Geometry check sheet. Reference: the model listing, model coordinates, mm. Give positions to 0.01 mm unless a question says otherwise; leave off trailing zeros. Write each loop counter-clockwise with the first axis right and the second up, starting at its lowest first coordinate (ties: lowest second). Pieces come first, ordered by that corner, then holes.
(1) Cross-section at B-B (z = -70). Record the boundary of the cut face in (x, y).
(2) Depth check by flat-ended pin: P1, Ø4, axis at y = 188, z = -296, coming from the -X side. Enter the tip coordinate at first touch or a pass-through.
(3) Cross-section at A-A (y = 65). Record the boundary of the cut face in (x, z).
(4) Thickness scan on line 1 along Z through (x, y) = (0.6, 265.06); line 2 along Z through (x, y) = (0.55, 188); line 3 along Y through (x, z) = (0.5, -314). Record the ranges inside material, lowest first.
(5) Cross-section at C-C (x = 0.8). Count the separate pieces of the cut face and the enclosed holes in it, and give its area (3 significant figures).
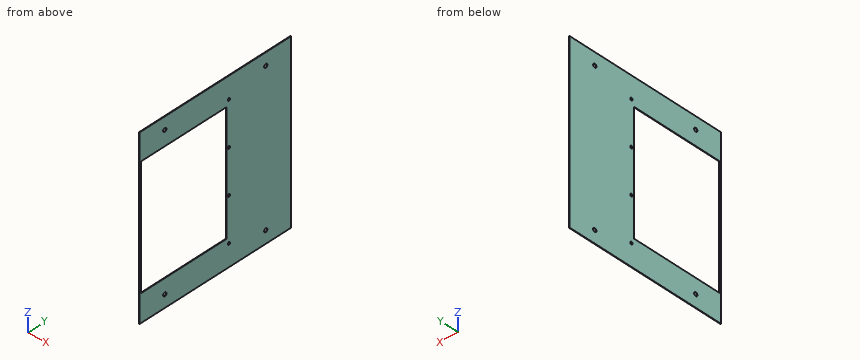
```python
from build123d import *

# Parameters (mm, degrees)
SKETCH1_W           = 338
SKETCH1_H           = 318
SKETCH1_R           = 3.5
BOSS_EXTRUDE1_DEPTH = 1
SKETCH2_R           = 2.5
SKETCH2_W           = 232.5
SKETCH2_H           = 180
CUT_EXTRUDE1_DEPTH  = 2


with BuildPart() as part:
    # Sketch1 → Boss-Extrude1 (new body)
    with BuildSketch(Plane(origin=(0, 0, 0), x_dir=(0, 0, -1), z_dir=(1, 0, 0))):
        with Locations((169, 159)):
            Rectangle(SKETCH1_W, SKETCH1_H)
        with Locations((24, 265.06)):
            Circle(SKETCH1_R, mode=Mode.SUBTRACT)
        with Locations((314, 265.06)):
            Circle(SKETCH1_R, mode=Mode.SUBTRACT)
        with Locations((314, 52.94)):
            Circle(SKETCH1_R, mode=Mode.SUBTRACT)
        with Locations((24, 52.94)):
            Circle(SKETCH1_R, mode=Mode.SUBTRACT)
    extrude(amount=BOSS_EXTRUDE1_DEPTH)

    # Sketch2 → Cut-Extrude1 (cut, through all)
    with BuildSketch(Plane.ZY):
        with Locations((-296, 188)):
            Circle(SKETCH2_R)
        with Locations((-211.333333333, 188)):
            Circle(SKETCH2_R)
        with Locations((-126.666666667, 188)):
            Circle(SKETCH2_R)
        with Locations((-42, 188)):
            Circle(SKETCH2_R)
        with Locations((-169, 93)):
            Rectangle(SKETCH2_W, SKETCH2_H)
    extrude(amount=-CUT_EXTRUDE1_DEPTH, mode=Mode.SUBTRACT)


solid = part.part
```
Reply:
1. outline: (0, 0) - (1, 0) - (1, 3) - (0, 3) - close; (0, 183) - (1, 183) - (1, 318) - (0, 318) - close
2. P1: passes through
3. outline: (0, -338) - (1, -338) - (1, -285.25) - (0, -285.25) - close; (0, -52.75) - (1, -52.75) - (1, 0) - (0, 0) - close
4. line 1: z = -338 to -317.5, -310.5 to -27.5, -20.5 to 0
4. line 2: z = -338 to -298.5, -293.5 to -213.83, -208.83 to -129.17, -124.17 to -44.5, -39.5 to 0
4. line 3: y = 0 to 49.44, 56.44 to 261.56, 268.56 to 318
5. separate pieces: 1
5. enclosed holes: 9
5. area: 65,400 mm2
